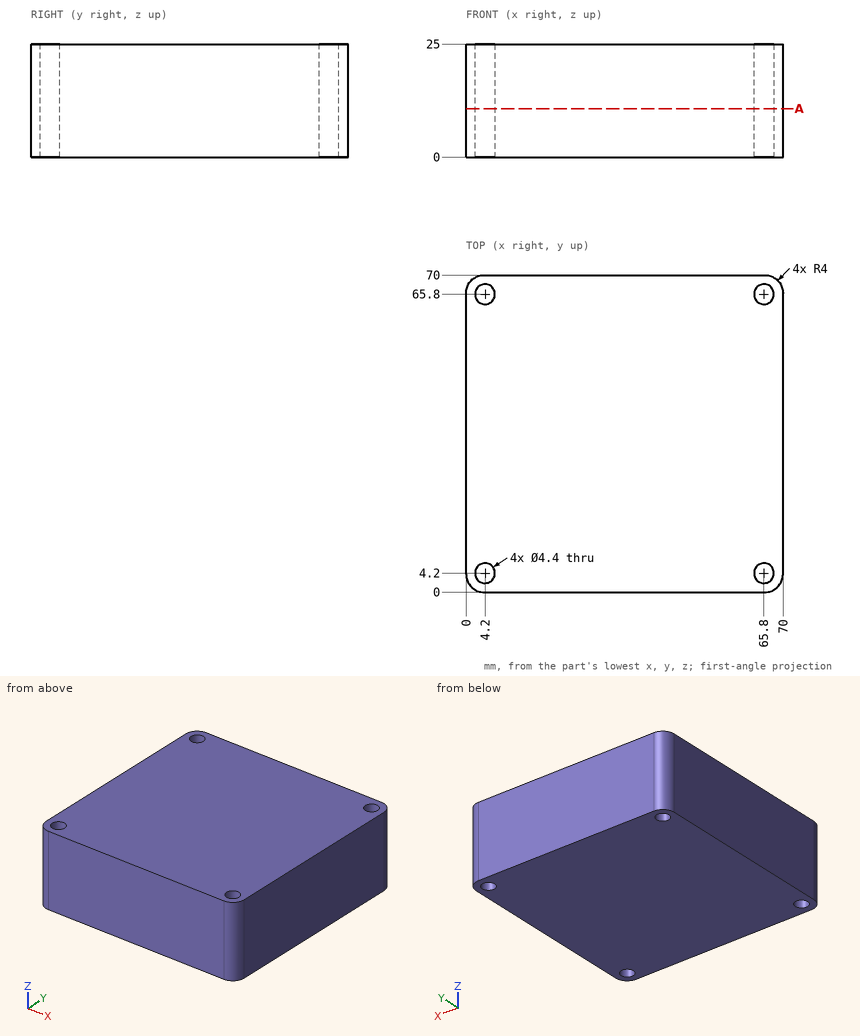
Here's the drawing with two shaded views (mm, measured from the low corner). I have some questions. Round coordinates to 2 decimals unless told otherwise and drop trailing zeros. Loops run counter-clockwise (first coordinate to the right, second up) from the corner with the lowest first, then second, coordinate; pieces in that order, holes last. Notation, with made-up numbers: (53.5, -15) - (106.5, -15) arc R18 ccw to (106.5, -1) - close; hole circle Ø2 at (53, 23). An arc over 180 degrees is marked (long way). Write item = value, one per line.
1) I'm going to push a flat-ended pin straight in: P1, Ø6, axis at y = 19.5, z = 16, coming from the -X side. Where does the tip first touch, or does it pass through?
Computed:
P1 = 0
2) I need wall thicknesses on line 1 along Y through (x, z) = (4.2, 15); line 2 along X through (y, z) = (66, 2.25); line 3 along X through (y, z) = (65, 11.25). Which ranges of each line are inside material? Lowest first, please. Write a range as from..to.
Computed:
line_1 = 0..2, 6.4..63.6, 68..70
line_2 = 0..2.01, 6.39..63.61, 67.99..70
line_3 = 0..2.15, 6.25..63.75, 67.85..70
3) Imagine slicing it at A-A (z = 10.75). Please give me the cut outline in (x, y), and give its area (3 significant figures).
Computed:
outline = (0, 4) arc R4 ccw to (4, 0) - (66, 0) arc R4 ccw to (70, 4) - (70, 66) arc R4 ccw to (66, 70) - (4, 70) arc R4 ccw to (0, 66) - close; hole circle Ø4.4 at (4.2, 4.2); hole circle Ø4.4 at (4.2, 65.8); hole circle Ø4.4 at (65.8, 4.2); hole circle Ø4.4 at (65.8, 65.8)
area = 4,830 mm2
